Input: part model. Units: mm. Frame: model coordinates. A direction names the side the tool comes from. Round coordinates to 2 decimals unless told otherwise and drop trailing zeros. Write each loop counter-clockwise with the first axis right and the second up, starting at its lowest first coordinate (ties: lowest second). Pieces come first, ordered by that corner, then holes. Notation, with made-up numbers: M -32,-36 L -13,-36 A21 ccw -13,-27 Z; hole C -7,-30 d11. An arc over 180 degrees is marked long. Answer as CSV lines item,"result". Start each with the question number.
```python
from build123d import *

# Parameters (mm, degrees)
SKETCH1_R                 = 3
CRANK_BODY_DEPTH          = 10
SKETCH2_R                 = 1.65
DOWEL_SHAFT_DEPTH         = 9
SKETCH3_R                 = 4.5
SKETCH3_W                 = 6
SKETCH3_H                 = 0.5
PIN_SHAFT_BODY_DEPTH      = 2
PIN_SHAFT_BODY_DEPTH_BACK = 2
SKETCH4_R                 = 2.5
PIN_SHAFT_DEPTH           = 6
SKETCH1_2_OUTSIDE_W       = 12.286
SKETCH1_2_OUTSIDE_H       = 15.286
SKETCH1_2_OUTSIDE_R       = 3
SMOOTHING_CUTS_DEPTH      = 10.5


with BuildPart() as part:
    # Sketch1 → crank_body (new body)
    with BuildSketch(Plane(origin=(0, 0, 0), x_dir=(1, 0, 0), z_dir=(0, 1, 0))):
        Circle(SKETCH1_R)
    extrude(amount=CRANK_BODY_DEPTH)

    # Sketch2 → dowel_shaft (cut)
    with BuildSketch(Plane.XZ):
        Circle(SKETCH2_R)
    extrude(amount=-DOWEL_SHAFT_DEPTH, mode=Mode.SUBTRACT)

    # Sketch3 → pin_shaft_body (add, two sides)
    with BuildSketch(Plane(origin=(0, 0, 0), x_dir=(0, 0, -1), z_dir=(1, 0, 0))) as pin_shaft_body_sk:
        with Locations((0, 14)):
            Circle(SKETCH3_R)
        with Locations((0, 10.25)):
            Rectangle(SKETCH3_W, SKETCH3_H)
    extrude(amount=PIN_SHAFT_BODY_DEPTH)
    extrude(pin_shaft_body_sk.sketch, amount=-PIN_SHAFT_BODY_DEPTH_BACK)

    # Sketch4 → pin_shaft (cut, through all)
    with BuildSketch(Plane(origin=(2, 0, 0), x_dir=(0, 0, -1), z_dir=(1, 0, 0))):
        with Locations((0, 14)):
            Circle(SKETCH4_R)
    extrude(amount=-PIN_SHAFT_DEPTH, mode=Mode.SUBTRACT)

    # Sketch1_2 outside → smoothing_cuts (cut)
    with BuildSketch(Plane(origin=(0, 0, 0), x_dir=(1, 0, 0), z_dir=(0, 1, 0))):
        Rectangle(SKETCH1_2_OUTSIDE_W, SKETCH1_2_OUTSIDE_H)
        Circle(SKETCH1_2_OUTSIDE_R, mode=Mode.SUBTRACT)
    extrude(amount=SMOOTHING_CUTS_DEPTH, mode=Mode.SUBTRACT)


solid = part.part
```
Item 1: Line query: line 1 (Y direction, x = 0.2, z = 0); line 2 (Z direction, x = 0, y = 6.25); line 3 (X direction, y = 8, z = 0.5). Output: solid intervals per line, ascending. Write a range as [from, to].
Item 2: Cut plane D-D, the plane y = 16. Return loops of the section in (x, z).
Item 3: Draft query along X for faces 1 (the face through (2, 12, 2)), 2 (the face through (-1.216, 4.437, 1.115)), 3 (the face through (2.4, 10, 0)). Return one class per face: +X half, -X half, draft (parallel to the pull), parting line (faces both ways), or undercut.
Item 4: Access query for faces 4 (the face through (-2, 12, 2)), 5 (the face through (0.03, 11.56, 0.54)), 6 (the face through (-3, 5, 0)). Directions: +Z, -Z, +X, -X, +Y, -Y. A direction counts if a zero-diameter tool reaches every point of the face in a straight line with its end or side. Return the directions, or none.
Item 5: Cut plane B-B, the plane z = 1. Return loops of the section in (x, y).
Item 6: Cut plane A-A, the plane x = 0. Return loops of the section in (y, z).
Item 7: Pin query (flat end, axial travel): pin 1 Ø3 at (y, z) = (14, 0) entering from +X; pin 2 Ø3 at (y, z) = (12, -1.5) entering from +X; pin 3 Ø1.5 at (x, z) = (2, 3) entering from +Y; pin 4 Ø1.1 at (x, z) = (2.5, -1) entering from +Y. Return the tip coordinate at first contact, or that it passes through.
Item 8: Cut plane C-C, the plane y = 14. Return loops of the section in (x, z), plus the area to 3 significant figures.
Results list:
1,line 1,"[9, 11.5], [16.5, 18.5]"
1,line 2,"[-3, -1.65], [1.65, 3]"
1,line 3,"[-2.96, -1.57], [1.57, 2.96]"
2,outline,"M -2,-4.03 L 2,-4.03 L 2,-1.5 L -2,-1.5 Z; M -2,1.5 L 2,1.5 L 2,4.03 L -2,4.03 Z"
3,face 1,"+X half"
3,face 2,"undercut"
3,face 3,"draft"
4,face 4,"+Z, -Z, -X, +Y"
4,face 5,"+X, -X"
4,face 6,"-Y"
5,outline,"M -2.83,0 L -1.31,0 L -1.31,9 L 1.31,9 L 1.31,0 L 2.83,0 L 2.83,10 L 2,10 L 2,11.71 L -2,11.71 L -2,10 L -2.83,10 Z; M -2,16.29 L 2,16.29 L 2,18.39 L -2,18.39 Z"
6,outline,"M 0,-3 L 10.5,-3 L 10.5,-2.83 A4.5 ccw long 10.5,2.83 L 10.5,3 L 0,3 L 0,1.65 L 9,1.65 L 9,-1.65 L 0,-1.65 Z; hole C 14,0 d5"
7,pin 1,"through"
7,pin 2,"x = 2"
7,pin 3,"y = 17.9"
7,pin 4,"y = 18.43"
8,outline,"M -2,-4.5 L 2,-4.5 L 2,-2.5 L -2,-2.5 Z; M -2,2.5 L 2,2.5 L 2,4.5 L -2,4.5 Z"
8,area,"16.0 mm²"
